Autodesk Inventor part; units mm, degrees
ref_plane "WeldJoint" through (0, 0, -10) normal (0.5, -0.866, 0) x (0, 0, 1)
ref_plane "Inlet_Clock_Angle_plane" through (0, 0, -10) normal (0, 1, 0) x (0, 0, 1)
ref_plane "Charging" through (0, 0, -10) normal (1, 0, 0) x (0, 0, 1)
sketch "Sketch13" plane through (0, 0, 0) normal (0, 0, 1) x (1, 0, 0)
  circle A0 centre (0, 0) radius 600 construction
  line L0 (0, 0) -> (0, -600)
  line L1 (0, 0) -> (-519.6152, -300)
  line L2 (0, 0) -> (600, 0)
  line L3 (0, 0) -> (0, -600)
  line L4 (0, 0) -> (0, -600)
  line L5 (0, 0) -> (534.6039, 272.3943)
  line L6 (0, 0) -> (0, 600)
  dimension "d53" = 1200
  dimension "d55" = 0
  dimension "d98" = 180
  dimension "d99" = 240
  dimension "d100" = 63
  dimension "d101" = 90
ref_plane "WeldJoint" through (0, 0, -10) normal (0.5, -0.866, 0) x (0, 0, 1)
ref_plane "Inlet_Clock_Angle_plane" through (0, 0, -10) normal (0, 1, 0) x (0, 0, 1)
ref_plane "Charging" through (0, 0, -10) normal (1, 0, 0) x (0, 0, 1)
ref_plane "Accsess" through (0, 0, -10) normal (1, 0, 0) x (0, 0, 1)
sketch "Sketch14" plane through (0, 0, -10) normal (0.5, -0.866, 0) x (0, 0, 1)
  line L0 (1510, 594) -> (10, 594)
  line L1 (10, 594) -> (10, 600)
  line L2 (10, 600) -> (1510, 600)
  line L3 (1510, 600) -> (1510, 594)
  line L4 (10, 0) -> (1510, 0)
  line L5 (10, 600) -> (-20, 600) construction
  line L6 (10, 594) -> (-20, 594) construction
  arc A0 (-20, 594) -> (-109.2789, 539.0476) centre (-20, 494) ccw construction
  arc A1 (-109.2789, 539.0476) -> (-234, 15) centre (929.3202, 15) ccw construction
  line L7 (-234, 15) -> (-234, 0) construction
  line L8 (10, 0) -> (-234, 0) construction
  arc A2 (-20, 600) -> (-114.6356, 541.7504) centre (-20, 494) ccw construction
  arc A3 (-114.6356, 541.7504) -> (-240, 15) centre (929.3202, 15) ccw construction
  line L9 (-240, 15) -> (-240, 0) construction
  line L10 (-234, 0) -> (-240, 0) construction
  line L11 (1510, 594) -> (1540, 594)
  line L12 (1510, 600) -> (1540, 600)
  line L13 (1510, 0) -> (1754, 0) construction
  line L14 (1760, 0) -> (1760, 15) construction
  arc A4 (1760, 15) -> (1634.6356, 541.7504) centre (590.6798, 15) ccw construction
  arc A5 (1634.6356, 541.7504) -> (1540, 600) centre (1540, 494) ccw construction
  line L15 (1754, 0) -> (1754, 15) construction
  line L16 (1754, 0) -> (1760, 0) construction
  arc A6 (1754, 15) -> (1629.2789, 539.0476) centre (590.6798, 15) ccw construction
  arc A7 (1629.2789, 539.0476) -> (1540, 594) centre (1540, 494) ccw construction
  line L17 (-156.8588, 530) -> (-610, 530)
  line L18 (-610, 530) -> (-610, 450)
  line L19 (-610, 450) -> (-156.8588, 450)
  line L20 (-156.8588, 450) -> (-156.8588, 530)
  line L21 (1760, 15) -> (1790, 15) construction
  line L22 (1790, 15) -> (1790, 0) construction
  line L23 (1790, 0) -> (1760, 0) construction
  line L24 (-610, 610) -> (-610, 530)
  line L25 (-610, 610) -> (-604, 610)
  line L26 (-604, 610) -> (-604, 530)
  line L27 (-115.4356, 543.7196) -> (-164.9441, 431.7071)
  line L28 (-156.8588, 530) -> (-121.4996, 530)
  line L29 (-109.2789, 539.0476) -> (-114.6356, 541.7504)
  line L30 (-115.4356, 543.7196) -> (-116.0014, 542.4396) construction
  line L31 (-116.0014, 542.4396) -> (-114.6356, 541.7504) construction
  point P0 (10, 597)
  point P1 (-140.1899, 487.7134)
  dimension "d59" = 1500
  dimension "d60" = 6
  dimension "d61" = 1200
  dimension "d82" = 100
  dimension "d83" = 30
  dimension "d86" = 80
  dimension "d87" = 30
  dimension "d88" = 2400
  dimension "d90" = 900
  dimension "d91" = 15
  dimension "d92" = 20
  dimension "d93" = 250
  dimension "d94" = 30
revolve "Revolution2" add sketch "Sketch14" angle 359.9 about axis through (0, 0, 0) along (0, 0, 1) contours L0 L1 L2 L3
sketch "Sketch AnglePlane_InletPipe" plane through (0, 0, -10) normal (0, 1, 0) x (0, 0, 1)
  line L0 (10, -600) -> (10, 600)
  line L1 (10, 0) -> (1310, 0)
  line L2 (1310, 0) -> (1310, 600)
  line L3 (1310, 600) -> (10, 600)
  line L4 (10, 600) -> (10, 0)
  point P0 (10, -519.6152)
  point P1 (10, -520.138)
  dimension "d63" = 1200
  dimension "d64" = 90
  dimension "frd_hght" = 1300
ref_plane "InletPipe_AnglePlane" through (0, 0, 1300) normal (1, 0, 0) x (0, 1, 0)
sketch "Sketch16" plane through (0, 0, 1300) normal (1, 0, 0) x (0, 1, 0)
  circle A0 centre (0, 0) radius 45.5
  point P0 (0, -1300)
  point P1 (0, 0)
  point P2 (0, 0)
  point P3 (0, 0)
  dimension "d66" = 91
extrude "Extrusion7" cut sketch "Sketch16" along normal through all
ref_plane "Work Plane16" through (0, 0, 0) normal (0, -1, 0) x (1, 0, 0)
sketch "Sketch17" plane through (0, 0, 0) normal (0, -1, 0) x (1, 0, 0)
  circle A0 centre (0, 408.5) radius 268.5
  line L0 (0, 140) -> (-495.5727, 140)
  point P0 (0, 0)
  dimension "d69" = 537
  dimension "d71" = 140
extrude "Extrusion8" cut sketch "Sketch17" along normal through all
sketch "Sketch19" plane through (0, 0, -10) normal (1, 0, 0) x (0, 0, 1)
  line L0 (10, 0) -> (1260, 0)
  line L1 (1260, 0) -> (1260, 600)
  line L2 (1260, 600) -> (10, 600)
  line L3 (10, 600) -> (10, 0)
  dimension "d74" = 1250
  dimension "d76" = 1200
  dimension "d77" = 90
ref_plane "Work Plane18" through (0, 0, 1250) normal (0, -1, 0) x (1, 0, 0)
sketch "Sketch20" plane through (0, 0, 1250) normal (0, -1, 0) x (1, 0, 0)
  line L0 (-103.5, 0) -> (103.5, 0)
  line L1 (103.5, 0) -> (103.5, 125)
  line L2 (103.5, 125) -> (-103.5, 125)
  line L3 (-103.5, 125) -> (-103.5, 0)
  point P0 (0, -1250)
  point P1 (0, 0)
  point P2 (0, 0)
  point P3 (0, 0)
  point P4 (0, 0)
  dimension "d78" = 207
  dimension "d79" = 125
extrude "Extrusion9" cut sketch "Sketch20" along normal through all
equation "\"BendRadius\" = Thickness"
equation "\"BendReliefWidth\" = Thickness"
equation "\"BendReliefDepth\" = 0.5 * Thickness"
equation "\"CornerReliefSize\" = 4 * Thickness"
equation "\"MinimumRemnant\" = 2 * Thickness"
equation "\"TransitionRadius\" = BendRadius"
equation "\"JacobiRadiusSize\" = BendRadius"
equation "\"GapSize\" = Thickness"
equation "\"InletPipe_horisont_angle\" = 0"
equation "\"AccsessHatch_diameter\" = 535"
equation "\"AccsessHatch_ClockAngle\" = 0"
equation "\"ChargingHatch_ClockAgnle\" = 180deg"
equation "\"InletPipe_Clock_angle\" = 90deg"
equation "\"OutletPipe_ClockAngle\" = 63deg"
equation "\"WeldJoint_ClockAgnle\" = 240deg"
properties part number "PRS 000 Filter1200 MAIN Shell" material "Steel"
The listing builds one solid part. Answer for the finished solid, in the listing's coordinates (mm). A direction names the side the tool comes from. Give positions to 0.01 mm unless a question says otherwise; leave off trailing zeros. Loops run counter-clockwise (first coordinate to the right, second up) from the corner with the lowest first, then second, coordinate; pieces in that order, holes last. Notation, with made-up numbers: (69.25, 70.25) - (121.25, 70.25) arc R33 ccw to (121.25, 101.25) - close; hole circle Ø8 at (-14.75, -38). An arc over 180 degrees is marked (long way). Write each question's results on one line, items separated by ' | '.
1. Find section C-C, the plane z = 408.5. Write down the section's boundary in (x, y).
Resolved:
outline: (-520.14, -299.09) - (-514.94, -296.1) arc R594 cw (long way) to (268.5, -529.85) - (268.5, -536.57) arc R600 ccw (long way) to start; (-519.62, -300) arc R600 ccw to (-268.5, -536.57) - (-268.5, -529.85) arc R594 cw to (-514.42, -297) - close
2. Flat-ended cylindrical pins translate along their axes: P1, Ø1, axis at x = 365.5, z = 1100, coming from the +Y side; P2, Ø6, axis at x = -432.5, z = 324.5, coming from the -Y side; P3, Ø1, axis at x = 379.5, z = 1329.5, coming from the +Y side. Find the tip coordinate at first contact, or state that the pin passes through.
Resolved:
P1: stops at y = 476.21 | P2: stops at y = -418.96 | P3: stops at y = 465.14
3. Consider probe 1 along Y at (x, z) = (0, 1045); probe 2 along Y at (x, z) = (73.5, 1437.5). Determine where each line is inside the solid, lowest interval first. Write a range as from..to.
Resolved:
probe 1: y = -600..-594, 594..600 | probe 2: y = -595.48..-589.44, 589.44..595.48
4. Find section B-B, the plane y = 0. Write down the section's boundary in (x, z), then the cut area to 3 significant figures.
Resolved:
outline: (-600, 0) - (-594, 0) - (-594, 1500) - (-600, 1500) - close; (594, 0) - (600, 0) - (600, 1254.5) - (594, 1254.5) - close; (594, 1345.5) - (600, 1345.5) - (600, 1500) - (594, 1500) - close | area: 17,500 mm^2
5. Which of the six approach directions +Z, -Z, +X, -X, +Y, -Y give full straight-line access (tool end or side, diameter ignored) to faces 4 (the face through (181.373, -567.36, 606.48)), 5 (the face through (571, 172, 0))?
Resolved:
face 4: -Y | face 5: -Z, +X, -X, +Y, -Y
6. For a pull along X with two mould halves and no side action, classify faces 1 (the face through (230.4, 554, 760.5)), 2 (the face through (596.073, -36.107, 1327.686)), 3 (the face through (179.03, 566.38, 739.5)) as +X half, -X half, draft (parallel to the pull), parting line (faces both ways), or undercut.
Resolved:
face 1: parting line | face 2: draft | face 3: undercut
7. Find section A-A, the plane x = 0. Write down the section's boundary in (y, z), then the cut area to 3 significant figures.
Resolved:
outline: (-600, 0) - (-594, 0) - (-594, 140) - (-600, 140) - close; (-600, 677) - (-594, 677) - (-594, 1250) - (-600, 1250) - close; (-600, 1375) - (-594, 1375) - (-594, 1500) - (-600, 1500) - close; (594, 0) - (600, 0) - (600, 1500) - (594, 1500) - close | area: 14,000 mm^2
